Verification items for the finished model (mm, model axes). A direction names the side the tool comes from. Give positions to 0.01 mm unless a question says otherwise; leave off trailing zeros. Order: outer loops, then holes, each group sorted by start corner. A loop starts at its lowest first (then second) coordinate and runs counter-clockwise, first axis right, second up. Notation, with made-up numbers: (81, 63.5) - (104, 63.5) arc R30 ccw to (104, 99.5) - close; hole circle Ø3 at (51.25, 26.25). An arc over 180 degrees is marked (long way). Answer as a JSON object with one key per item and string values. Group by question number.
(1) Section check A-A (x = 39). Record the boundary of the cut face in (y, z), then the cut area to 3 significant figures.
(2) Mould release check, pull along Z, two halves, no side actions. Record for faces 4 (the face through (70, -5, 20)), 5 (the face through (20.2, -5.07, 21.95)), 6 (the face through (35, -5, 0)), 7 (the face through (35, -5, 40)): +Z half, -Z half, draft (parallel to the pull), parting line (faces both ways), or undercut.
(3) Section check C-C (x = 14). Record the boundary of the cut face in (y, z).
(4) Access from +Z, -Z, +X, -X, +Y, -Y to the whole of each face (thin tool, end or side, straight path). Record for faces 1 (the face through (3.98, -3.87, 21.77)), 2 (the face through (35, -10, 20)), 3 (the face through (3.7, -5.1, 6.1)).
(5) Section check B-B (y = -8). Record the boundary of the cut face in (x, z).
(6) Thickness scan on line 1 (Z direction, x = 7, y = -7.25); line 2 (Z direction, x = 5, y = -5); line 3 (Y direction, x = 5, z = 20). Record the ranges inside material, lowest first.
(7) Depth check by flat-ended pin: pin 1 Ø17 at (x, z) = (14, 20) entering from +Y. Enter the tip coordinate at first touch or a pass-through.
(8) Section check D-D (z = 16.5). Record the boundary of the cut face in (x, y), then the cut area to 3 significant figures.
```python
from build123d import *

# Parameters (mm, degrees)
F0_W     = 70
F0_H     = 40
F1_DEPTH = 10
F2_R     = 6.5
F3_DEPTH = 25
F5_D     = 4.2
F5_DEPTH = 15
F5_TIP   = 1.2618073


with BuildPart() as f1:
    # F0 (on Front) → F1 (new body)
    with BuildSketch(Plane.XZ):
        with Locations((35, 20)):
            Rectangle(F0_W, F0_H)
    extrude(amount=F1_DEPTH)

    # F2 (on face) → F3 (cut)
    with BuildSketch(Plane.XZ.offset(10)):
        with BuildLine():
            Line((62, 30.7), (62, 37.3))
            ThreePointArc((62, 37.3), (58.7, 34), (62, 30.7))
        make_face()
        with BuildLine():
            ThreePointArc((62, 30.7), (64.3334523779, 31.6665476221), (65.3, 34))
            ThreePointArc((65.3, 34), (64.3334523779, 36.3334523779), (62, 37.3))
            Line((62, 37.3), (62, 30.7))
        make_face()
        with BuildLine():
            ThreePointArc((10.3, 34), (9.3334523779, 36.3334523779), (7, 37.3))
            ThreePointArc((7, 37.3), (3.7, 34), (7, 30.7))
            ThreePointArc((7, 30.7), (9.3334523779, 31.6665476221), (10.3, 34))
        make_face()
        with BuildLine():
            ThreePointArc((7, 2.7), (9.3334523779, 3.6665476221), (10.3, 6))
            ThreePointArc((10.3, 6), (9.3334523779, 8.3334523779), (7, 9.3))
            ThreePointArc((7, 9.3), (3.7, 6), (7, 2.7))
        make_face()
        with BuildLine():
            Line((62, 2.7), (62, 9.3))
            ThreePointArc((62, 9.3), (58.7, 6), (62, 2.7))
        make_face()
        with BuildLine():
            ThreePointArc((65.3, 6), (64.3334523779, 8.3334523779), (62, 9.3))
            Line((62, 9.3), (62, 2.7))
            ThreePointArc((62, 2.7), (64.3334523779, 3.6665476221), (65.3, 6))
        make_face()
        with BuildLine():
            ThreePointArc((62, 30.7), (58.7, 34), (62, 37.3))
            Line((62, 37.3), (7, 37.3))
            ThreePointArc((7, 37.3), (9.3334523779, 36.3334523779), (10.3, 34))
            ThreePointArc((10.3, 34), (9.3334523779, 31.6665476221), (7, 30.7))
            Line((7, 30.7), (62, 30.7))
        make_face()
        with BuildLine():
            ThreePointArc((7, 9.3), (9.3334523779, 8.3334523779), (10.3, 6))
            ThreePointArc((10.3, 6), (9.3334523779, 3.6665476221), (7, 2.7))
            Line((7, 2.7), (62, 2.7))
            ThreePointArc((62, 2.7), (58.7, 6), (62, 9.3))
            Line((62, 9.3), (7, 9.3))
        make_face()
        with Locations((14, 20)):
            Circle(F2_R)
    extrude(amount=-F3_DEPTH, mode=Mode.SUBTRACT)

    # F5
    with Locations(Plane(origin=(0, 0, 0), x_dir=(0, -1, 0), z_dir=(-1, 0, 0))):
        with Locations((5, 20)):
            Hole(F5_D / 2, depth=F5_DEPTH)
            with Locations((0, 0, -(F5_DEPTH + F5_TIP / 2))):  # 118° drill point
                Cone(0, F5_D / 2, F5_TIP, mode=Mode.SUBTRACT)


solid = f1.part
```
Solutions:
{
 "1": {"outline": "(-10, 0) - (0, 0) - (0, 2.7) - (-10, 2.7) - close; (-10, 9.3) - (0, 9.3) - (0, 30.7) - (-10, 30.7) - close; (-10, 37.3) - (0, 37.3) - (0, 40) - (-10, 40) - close", "area": "268 mm2"},
 "2": {"face 4": "draft", "face 5": "undercut", "face 6": "-Z half", "face 7": "+Z half"},
 "3": {"outline": "(-10, 0) - (0, 0) - (0, 2.7) - (-10, 2.7) - close; (-10, 9.3) - (0, 9.3) - (0, 13.5) - (-10, 13.5) - close; (-10, 26.5) - (0, 26.5) - (0, 30.7) - (-10, 30.7) - close; (-10, 37.3) - (0, 37.3) - (0, 40) - (-10, 40) - close"},
 "4": {"face 1": "-X", "face 2": "+Z, -Z, +X, -X, -Y", "face 3": "+Y, -Y"},
 "5": {"outline": "(0, 0) - (70, 0) - (70, 40) - (0, 40) - close; hole (7, 2.7) - (62, 2.7) arc R3.3 ccw to (62, 9.3) - (7, 9.3) arc R3.3 ccw to start; hole (7, 30.7) - (62, 30.7) arc R3.3 ccw to (62, 37.3) - (7, 37.3) arc R3.3 ccw to start; hole circle Ø13 at (14, 20)"},
 "6": {"line 1": "z = 0 to 2.7, 9.3 to 30.7, 37.3 to 40", "line 2": "z = 0 to 3.38, 8.62 to 17.9, 22.1 to 31.38, 36.62 to 40", "line 3": "y = -10 to -7.1, -2.9 to 0"},
 "7": {"pin 1": "stops at y = 0"},
 "8": {"outline": "(0, -10) - (8.52, -10) - (8.52, 0) - (0, 0) - close; (19.48, -10) - (70, -10) - (70, 0) - (19.48, 0) - close", "area": "590 mm2"}
}
